from build123d import *

# Parameters (mm, degrees)
SKETCH1_W           = 21
SKETCH1_H           = 51
TOPFACE_DEPTH       = 1
SKETCH2_R           = 0.5
SKETCH2_R_2         = 1
CUT_EXTRUDE1_DEPTH  = 28.595289453
SKETCH3_W           = 7
SKETCH3_H           = 7
BOSS_EXTRUDE2_DEPTH = 1
SKETCH4_W           = 3
SKETCH4_H           = 4
BOSS_EXTRUDE3_DEPTH = 2
BOSS_EXTRUDE4_DEPTH = 1
SKETCH6_W           = 1.5
SKETCH6_H           = 3
SKETCH6_W_2         = 2
SKETCH6_H_2         = 2.5
SKETCH6_W_3         = 2.5
SKETCH6_W_4         = 3
BOSS_EXTRUDE5_DEPTH = 1
SKETCH7_W           = 2.5
SKETCH7_H           = 1
BOSS_EXTRUDE6_DEPTH = 2
BOSS_EXTRUDE7_DEPTH = 4
BOSS_EXTRUDE8_START = 1
BOSS_EXTRUDE8_DEPTH = 1
CUT_EXTRUDE2_DEPTH  = 4.8
SKETCH11_W          = 3
SKETCH11_H          = 0.2
BOSS_EXTRUDE9_DEPTH = 3


with BuildPart() as part:
    # Sketch1 → TopFace (new body)
    with BuildSketch(Plane(origin=(0, 0, 0), x_dir=(1, 0, 0), z_dir=(0, 1, 0))):
        Rectangle(SKETCH1_W, SKETCH1_H)
    extrude(amount=TOPFACE_DEPTH)

    # Sketch2 → Cut-Extrude1 (cut, through all)
    with BuildSketch(Plane(origin=(0, 1, 0), x_dir=(1, 0, 0), z_dir=(0, 1, 0))):
        with Locations(Location((-9, 23.75, 0), (0, 0, 270))):
            Circle(SKETCH2_R)
        with Locations(Location((-9, 21.25, 0), (0, 0, 270))):
            Circle(SKETCH2_R)
        with Locations(Location((-9, 18.75, 0), (0, 0, 270))):
            Circle(SKETCH2_R)
        with Locations(Location((-9, 16.25, 0), (0, 0, 270))):
            Circle(SKETCH2_R)
        with Locations(Location((-9, 13.75, 0), (0, 0, 270))):
            Circle(SKETCH2_R)
        with Locations(Location((-9, 11.25, 0), (0, 0, 270))):
            Circle(SKETCH2_R)
        with Locations(Location((-9, 8.75, 0), (0, 0, 270))):
            Circle(SKETCH2_R)
        with Locations(Location((-9, 6.25, 0), (0, 0, 270))):
            Circle(SKETCH2_R)
        with Locations(Location((-9, 3.75, 0), (0, 0, 270))):
            Circle(SKETCH2_R)
        with Locations(Location((-9, 1.25, 0), (0, 0, 270))):
            Circle(SKETCH2_R)
        with Locations(Location((-9, -1.25, 0), (0, 0, 270))):
            Circle(SKETCH2_R)
        with Locations(Location((-9, -3.75, 0), (0, 0, 270))):
            Circle(SKETCH2_R)
        with Locations(Location((-9, -6.25, 0), (0, 0, 270))):
            Circle(SKETCH2_R)
        with Locations(Location((-9, -8.75, 0), (0, 0, 270))):
            Circle(SKETCH2_R)
        with Locations(Location((-9, -11.25, 0), (0, 0, 270))):
            Circle(SKETCH2_R)
        with Locations(Location((-9, -13.75, 0), (0, 0, 270))):
            Circle(SKETCH2_R)
        with Locations(Location((-9, -16.25, 0), (0, 0, 270))):
            Circle(SKETCH2_R)
        with Locations(Location((-9, -18.75, 0), (0, 0, 270))):
            Circle(SKETCH2_R)
        with Locations(Location((-9, -21.25, 0), (0, 0, 270))):
            Circle(SKETCH2_R)
        with Locations(Location((-9, -23.75, 0), (0, 0, 270))):
            Circle(SKETCH2_R)
        with Locations(Location((9, -23.75, 0), (0, 0, 90))):
            Circle(SKETCH2_R)
        with Locations(Location((9, -21.25, 0), (0, 0, 90))):
            Circle(SKETCH2_R)
        with Locations(Location((9, -18.75, 0), (0, 0, 90))):
            Circle(SKETCH2_R)
        with Locations(Location((9, -16.25, 0), (0, 0, 90))):
            Circle(SKETCH2_R)
        with Locations(Location((9, -13.75, 0), (0, 0, 90))):
            Circle(SKETCH2_R)
        with Locations(Location((9, -11.25, 0), (0, 0, 90))):
            Circle(SKETCH2_R)
        with Locations(Location((9, -8.75, 0), (0, 0, 90))):
            Circle(SKETCH2_R)
        with Locations(Location((9, -6.25, 0), (0, 0, 90))):
            Circle(SKETCH2_R)
        with Locations(Location((9, -3.75, 0), (0, 0, 90))):
            Circle(SKETCH2_R)
        with Locations(Location((9, -1.25, 0), (0, 0, 90))):
            Circle(SKETCH2_R)
        with Locations(Location((9, 1.25, 0), (0, 0, 90))):
            Circle(SKETCH2_R)
        with Locations(Location((9, 3.75, 0), (0, 0, 90))):
            Circle(SKETCH2_R)
        with Locations(Location((9, 6.25, 0), (0, 0, 90))):
            Circle(SKETCH2_R)
        with Locations(Location((9, 8.75, 0), (0, 0, 90))):
            Circle(SKETCH2_R)
        with Locations(Location((9, 11.25, 0), (0, 0, 90))):
            Circle(SKETCH2_R)
        with Locations(Location((9, 13.75, 0), (0, 0, 90))):
            Circle(SKETCH2_R)
        with Locations(Location((9, 16.25, 0), (0, 0, 90))):
            Circle(SKETCH2_R)
        with Locations(Location((9, 18.75, 0), (0, 0, 90))):
            Circle(SKETCH2_R)
        with Locations(Location((9, 21.25, 0), (0, 0, 90))):
            Circle(SKETCH2_R)
        with Locations(Location((9, 23.75, 0), (0, 0, 90))):
            Circle(SKETCH2_R)
        with Locations(Location((0, -23.5, 0), (0, 0, 270))):
            Circle(SKETCH2_R)
        with Locations(Location((-2.5, -23.5, 0), (0, 0, 270))):
            Circle(SKETCH2_R)
        with Locations(Location((2.5, -23.5, 0), (0, 0, 90))):
            Circle(SKETCH2_R)
        with Locations(Location((-5.5, -23.5, 0), (0, 0, 270))):
            Circle(SKETCH2_R_2)
        with Locations(Location((5.5, -23.5, 0), (0, 0, 90))):
            Circle(SKETCH2_R_2)
        with Locations(Location((-5.5, 23.5, 0), (0, 0, 90))):
            Circle(SKETCH2_R_2)
        with Locations(Location((5.5, 23.5, 0), (0, 0, 270))):
            Circle(SKETCH2_R_2)
    extrude(amount=-CUT_EXTRUDE1_DEPTH, mode=Mode.SUBTRACT)

    # Sketch3 → Boss-Extrude2 (add)
    with BuildSketch(Plane(origin=(0, 1, 0), x_dir=(1, 0, 0), z_dir=(0, 1, 0))):
        Rectangle(SKETCH3_W, SKETCH3_H)
    extrude(amount=BOSS_EXTRUDE2_DEPTH)

    # Sketch4 → Boss-Extrude3 (add)
    with BuildSketch(Plane(origin=(0, 1, 0), x_dir=(1, 0, 0), z_dir=(0, 1, 0))):
        with Locations((-3.5, 13.75)):
            Rectangle(SKETCH4_W, SKETCH4_H)
    extrude(amount=BOSS_EXTRUDE3_DEPTH)

    # Sketch5 → Boss-Extrude4 (add)
    with BuildSketch(Plane(origin=(0, 3, 0), x_dir=(1, 0, 0), z_dir=(0, 1, 0))):
        with BuildLine():
            Line((-2.5, 14.25), (-2.5, 13.25))
            ThreePointArc((-2.5, 13.25), (-3.5, 12.25), (-4.5, 13.25))
            Line((-4.5, 13.25), (-4.5, 14.25))
            ThreePointArc((-4.5, 14.25), (-3.5, 15.25), (-2.5, 14.25))
        make_face()
    extrude(amount=BOSS_EXTRUDE4_DEPTH)

    # Sketch6 → Boss-Extrude5 (add)
    with BuildSketch(Plane(origin=(0, 1, 0), x_dir=(1, 0, 0), z_dir=(0, 1, 0))):
        with Locations((7, 18.75)):
            Rectangle(SKETCH6_W, SKETCH6_H)
        with Locations((7, 14)):
            Rectangle(SKETCH6_W_2, SKETCH6_H_2)
        with Locations((3.75, 14)):
            Rectangle(SKETCH6_W_3, SKETCH6_H)
        with Locations((-4, 6.25)):
            Rectangle(SKETCH6_W_2, SKETCH6_H)
        with Locations((-2.5, -8.75)):
            Rectangle(SKETCH6_W_4, SKETCH6_H_2)
    extrude(amount=BOSS_EXTRUDE5_DEPTH)

    # Sketch7 → Boss-Extrude6 (add)
    with BuildSketch(Plane(origin=(0, 1, 0), x_dir=(1, 0, 0), z_dir=(0, 1, 0))):
        with Locations((3.75, 17)):
            Rectangle(SKETCH7_W, SKETCH7_H)
        with Locations((3.75, 11)):
            Rectangle(SKETCH7_W, SKETCH7_H)
    extrude(amount=BOSS_EXTRUDE6_DEPTH)

    # Sketch8 → Boss-Extrude7 (add)
    with BuildSketch(Plane(origin=(0, 0, -25.5), x_dir=(-1, 0, 0), z_dir=(0, 0, -1))):
        with BuildLine():
            Line((-3.25, 4), (3.25, 4))
            ThreePointArc((3.25, 4), (3.603553391, 3.853553391), (3.75, 3.5))
            Line((3.75, 3.5), (3.75, 3))
            ThreePointArc((3.75, 3), (3.164213562, 1.585786438), (1.75, 1))
            Line((1.75, 1), (-1.75, 1))
            ThreePointArc((-1.75, 1), (-3.164213562, 1.585786438), (-3.75, 3))
            Line((-3.75, 3), (-3.75, 3.5))
            ThreePointArc((-3.75, 3.5), (-3.603553391, 3.853553391), (-3.25, 4))
        make_face()
    extrude(amount=-BOSS_EXTRUDE7_DEPTH)

    # Sketch9 → Boss-Extrude8 (add)
    with BuildSketch(Plane(origin=(0, 0, -25.5), x_dir=(-1, 0, 0), z_dir=(0, 0, -1)).offset(BOSS_EXTRUDE8_START)):
        with BuildLine():
            Line((-1.75, 1), (1.75, 1))
            ThreePointArc((1.75, 1), (3.164213562, 1.585786438), (3.75, 3))
            Line((3.75, 3), (3.75, 3.5))
            ThreePointArc((3.75, 3.5), (3.603553391, 3.853553391), (3.25, 4))
            Line((3.25, 4), (-3.25, 4))
            ThreePointArc((-3.25, 4), (-3.603553391, 3.853553391), (-3.75, 3.5))
            Line((-3.75, 3.5), (-3.75, 3))
            ThreePointArc((-3.75, 3), (-3.164213562, 1.585786438), (-1.75, 1))
        make_face()
    extrude(amount=-BOSS_EXTRUDE8_DEPTH)

    # Sketch10 → Cut-Extrude2 (cut)
    with BuildSketch(Plane(origin=(0, 0, -26.5), x_dir=(-1, 0, 0), z_dir=(0, 0, -1))):
        with BuildLine():
            Line((3.25, 3.9), (-3.25, 3.9))
            ThreePointArc((-3.25, 3.9), (-3.532842712, 3.782842712), (-3.65, 3.5))
            Line((-3.65, 3.5), (-3.65, 3))
            ThreePointArc((-3.65, 3), (-3.093502884, 1.656497116), (-1.75, 1.1))
            Line((-1.75, 1.1), (1.75, 1.1))
            ThreePointArc((1.75, 1.1), (3.093502884, 1.656497116), (3.65, 3))
            Line((3.65, 3), (3.65, 3.5))
            ThreePointArc((3.65, 3.5), (3.532842712, 3.782842712), (3.25, 3.9))
        make_face()
    extrude(amount=-CUT_EXTRUDE2_DEPTH, mode=Mode.SUBTRACT)

    # Sketch11 → Boss-Extrude9 (add)
    with BuildSketch(Plane(origin=(0, 0, -21.7), x_dir=(-1, 0, 0), z_dir=(0, 0, -1))):
        with Locations((0, 3.15)):
            Rectangle(SKETCH11_W, SKETCH11_H)
    extrude(amount=BOSS_EXTRUDE9_DEPTH)


solid = part.part
Build history of the part. All positions in model axes, mm. A direction names the side the tool comes from. Round coordinates to 2 decimals unless told otherwise and drop trailing zeros. Write each loop counter-clockwise with the first axis right and the second up, starting at its lowest first coordinate (ties: lowest second). Pieces come first, ordered by that corner, then holes. Notation, with made-up numbers: (8.5, 17) -> (30.5, 17) arc R31 ccw to (30.5, 45) -> close; hole circle Ø5 at (31, -1.75). An arc over 180 degrees is marked (long way). Write item = value, one per line.
(1) Tool access for faces 1 (the face through (7.75, 1.5, -18.7)), 2 (the face through (4, 2, -11.5)), 3 (the face through (-2, 2, -14)): list every direction of +Z, -Z, +X, -X, +Y, -Y with a clear straight run to the whole face (end or side of a thin tool).
Answer:
face_1 = -Z, +X, +Y
face_2 = +X, -X, +Y
face_3 = +Y
(2) Band-saw the part on A-A (z = 11.25). Give the cut face in (x, y), then the cut area to 3 significant figures.
Answer:
outline = (-10.5, 0) -> (-9.5, 0) -> (-9.5, 1) -> (-10.5, 1) -> close; (-8.5, 0) -> (8.5, 0) -> (8.5, 1) -> (-8.5, 1) -> close; (9.5, 0) -> (10.5, 0) -> (10.5, 1) -> (9.5, 1) -> close
area = 19.0 mm2
(3) Band-saw the part on D-D (z = -18.75). Give the cut face in (x, y), then the cut area to 3 significant figures.
Answer:
outline = (-10.5, 0) -> (-9.5, 0) -> (-9.5, 1) -> (-10.5, 1) -> close; (-8.5, 0) -> (8.5, 0) -> (8.5, 1) -> (7.75, 1) -> (7.75, 2) -> (6.25, 2) -> (6.25, 1) -> (-8.5, 1) -> close; (9.5, 0) -> (10.5, 0) -> (10.5, 1) -> (9.5, 1) -> close
area = 20.5 mm2
(4) Band-saw the part on B-B (z = 2.5). Give the cut face in (x, y).
Answer:
outline = (-10.5, 0) -> (10.5, 0) -> (10.5, 1) -> (3.5, 1) -> (3.5, 2) -> (-3.5, 2) -> (-3.5, 1) -> (-10.5, 1) -> close
(5) Two-plate mould, pull along Z, no slides. Class faces 4 (the face through (-4.5, 3.5, -13.7)), 5 (the face through (-9.488, 0.507, 3.642)): pulls with the +Z half, pulls with the -Z half, needs draft (parallel to the pull), parting line crosses it, or undercut.
Answer:
face_4 = needs draft
face_5 = undercut
(6) Band-saw the part on C-C (x = 1). Give the cut face in (y, z).
Answer:
outline = (0, -25.5) -> (1, -25.5) -> (1, -26.5) -> (1.1, -26.5) -> (1.1, -21.7) -> (3.05, -21.7) -> (3.05, -24.7) -> (3.25, -24.7) -> (3.25, -21.7) -> (3.9, -21.7) -> (3.9, -26.5) -> (4, -26.5) -> (4, -21.5) -> (1, -21.5) -> (1, -3.5) -> (2, -3.5) -> (2, 3.5) -> (1, 3.5) -> (1, 25.5) -> (0, 25.5) -> close
(7) Probe L1, parallel to X at y = 0.5, z = -6.25; L2, parallel to Z at x = 7.25, y = 1.05; L3, parallel to Y at x = -7.75, z = 11.5. List the from-to ranges inside material, lowest first.
Answer:
L1 = -10.5 to -9.5, -8.5 to 8.5, 9.5 to 10.5
L2 = -20.25 to -17.25, -15.25 to -12.75
L3 = 0 to 1
(8) Flat gauge pins, fed straight in: pin 1 (0.8 mm diameter, centred on x = 3.5, z = -14.5, fed in from +Y); pin 2 (1.6 mm diameter, centred on x = 3.5, y = 2.5, fed in from +Z); pin 3 (2 mm diameter, centred on x = 4.5, y = 3, fed in from +Z). Where does each tip first touch, or does it go through?
Answer:
pin_1 = 2
pin_2 = 3.5
pin_3 = -10.5
